The listing builds one solid part. Answer for the finished solid, in the listing's coordinates (mm). Coordinates: 2 decimals unless noted, no trailing zeros. Write each loop counter-clockwise with the first axis right and the second up, starting at its lowest first coordinate (ties: lowest second). Pieces come first, ordered by that corner, then holes.
from build123d import *

# Parameters (mm, degrees)
BOSS_EXTRUDE1_DEPTH = 3.2
SKETCH11_W          = 3.2
SKETCH11_H          = 199.000000018
CUT_EXTRUDE1_DEPTH  = 284.232260808
SKETCH13_W          = 50.8
SKETCH13_H          = 54.36
CUT_EXTRUDE3_DEPTH  = 284.232260808


with BuildPart() as part:
    # Sketch1 → Boss-Extrude1 (new body)
    with BuildSketch(Plane(origin=(0, 0, 0), x_dir=(1, 0, 0), z_dir=(0, 1, 0))):
        Polygon((265.160373285, -79.687626629), (259.623773233, -79.687626629), (259.623773233, -81.450000041), (-255.462493265, -81.450000041), (-255.462493265, -79.687626629), (-260.999093317, -79.687626629), (-260.999093317, 99.500000009), (265.160373285, 99.500000009), align=None)
    extrude(amount=BOSS_EXTRUDE1_DEPTH)

    # Sketch11 → Cut-Extrude1 (cut, through all)
    with BuildSketch(Plane(origin=(0, 3.2, 0), x_dir=(1, 0, 0), z_dir=(0, 1, 0))):
        with Locations((2.080639984, 99.500000009)):
            Rectangle(SKETCH11_W, SKETCH11_H)
    extrude(amount=-CUT_EXTRUDE1_DEPTH, mode=Mode.SUBTRACT)

    # Sketch13 → Cut-Extrude3 (cut, through all)
    with BuildSketch(Plane(origin=(0, 3.2, 0), x_dir=(1, 0, 0), z_dir=(0, 1, 0))):
        with Locations((-24.919360016, 72.320000009)):
            Rectangle(SKETCH13_W, SKETCH13_H)
        with Locations((29.080639984, 72.320000009)):
            Rectangle(SKETCH13_W, SKETCH13_H)
    extrude(amount=-CUT_EXTRUDE3_DEPTH, mode=Mode.SUBTRACT)


solid = part.part
Q1. The part is cut by section A-A, the plane z = -73. Write down the section's boundary in (x, y).
Answers below:
outline: (-261, 0) - (-50.32, 0) - (-50.32, 3.2) - (-261, 3.2) - close; (54.48, 0) - (265.16, 0) - (265.16, 3.2) - (54.48, 3.2) - close
Q2. The part is cut by section C-C, the plane x = -14.5. Write down the section's boundary in (y, z), then the cut area to 3 significant figures.
Answers below:
outline: (0, -45.14) - (3.2, -45.14) - (3.2, 81.45) - (0, 81.45) - close
area: 405 mm2
Q3. Given pin 1 (0.5 mm diameter, centred on y = 1.5, z = 80.5, fed in from +X); pin 2 (1.6 mm diameter, centred on x = 2.5, y = 2, fed in from -Z); pin 3 (0.5 mm diameter, centred on y = 2.5, z = 81, fed in from -X), each flat-ended and moving along its own axis, determine where each tip first touches the part or whether it passes through.
Answers below:
pin 1: stops at x = 259.62
pin 2: stops at z = 0
pin 3: stops at x = -255.46
Q4. The part is cut by section B-B, the plane y = 2.5. Write down the section's boundary in (x, z), then the cut area to 3 significant figures.
Answers below:
outline: (-261, -99.5) - (-50.32, -99.5) - (-50.32, -45.14) - (0.48, -45.14) - (0.48, 0) - (3.68, 0) - (3.68, -45.14) - (54.48, -45.14) - (54.48, -99.5) - (265.16, -99.5) - (265.16, 79.69) - (259.62, 79.69) - (259.62, 81.45) - (-255.46, 81.45) - (-255.46, 79.69) - (-261, 79.69) - close
area: 89,300 mm2
Q5. Find the intervals of material crossed by probe 1 along X at (y, z) = (3, -62); probe 2 along X at (y, z) = (0.8, -39); probe 3 along Z at (x, y) = (-20, 0.75), in increasing order.
Answers below:
probe 1: x = -261 to -50.32, 54.48 to 265.16
probe 2: x = -261 to 0.48, 3.68 to 265.16
probe 3: z = -45.14 to 81.45
